```python
from build123d import *

# Parameters (mm, degrees)
SKETCH_2_W               = 1.6
SKETCH_2_H               = 0.7
CUT_EXTRUDE_1_DEPTH      = 3.5
CUT_EXTRUDE_1_DEPTH_BACK = 3.5
CHAMFER_1_SIZE           = 0.2


with BuildPart() as part:
    # 草图1 → 旋转1 (revolve)
    with BuildSketch(Plane(origin=(0, 0, 0), x_dir=(0, 0, -1), z_dir=(1, 0, 0))):
        Polygon((0, 0), (0, 2.5), (1.5, 2.5), (1.5, 1.5), (9.5, 1.5), (9.5, 0.7), (9.8, 0.7), (9.8, 1), (13.5, 1), (13.5, 0), align=None)
    revolve(axis=Axis((0, 0, -13.5), (0, 0, 1)))

    # 草图2 → 切除-拉伸1 (cut, two sides)
    with BuildSketch(Plane(origin=(0, 0, 0), x_dir=(0, 0, -1), z_dir=(1, 0, 0))) as cut_extrude_1_sk:
        Rectangle(SKETCH_2_W, SKETCH_2_H)
    extrude(amount=CUT_EXTRUDE_1_DEPTH, mode=Mode.SUBTRACT)
    extrude(cut_extrude_1_sk.sketch, amount=-CUT_EXTRUDE_1_DEPTH_BACK, mode=Mode.SUBTRACT)

    # 倒角1
    chamfer_1_edges = [part.edges().sort_by_distance(p)[0] for p in [
        (0, -2.5, 0),
        (-1.639359631, 1.887458609, 0),
    ]]
    chamfer(chamfer_1_edges, length=CHAMFER_1_SIZE)


solid = part.part
```
The model under review builds one solid part; all positions refer to its coordinate system, in mm. A direction names the side the tool comes from. Round coordinates to 2 decimals unless told otherwise and drop trailing zeros. Order: outer loops, then holes, each group sorted by start corner. A loop starts at its lowest first (then second) coordinate and runs counter-clockwise, first axis right, second up.
Item 1: Machinability: for faces 5 (the cylindrical face through (1, 0, -12)), 6 (the flat face through (0, 0, -13.5)), 7 (the flat face through (0, -0.35, -0.4)), which of the approach directions +Z, -Z, +X, -X, +Y, -Y give a long, thin tool a straight path to every point of the face, cutting with its end or side? Answer none if there is none.
Working result:
face 5: -Z
face 6: -Z, +X, -X, +Y, -Y
face 7: +Z, +X, -X
Item 2: Add section A-A, the plane y = 0. State the section outline as (x, z) points, and give its area (3 significant figures).
Working result:
outline: (-2.5, -1.5) - (-1.5, -1.5) - (-1.5, -9.5) - (-0.7, -9.5) - (-0.7, -9.8) - (-1, -9.8) - (-1, -13.5) - (1, -13.5) - (1, -9.8) - (0.7, -9.8) - (0.7, -9.5) - (1.5, -9.5) - (1.5, -1.5) - (2.5, -1.5) - (2.5, -0.8) - (-2.5, -0.8) - close
area: 35.3 mm2
Item 3: Add section C-C, the plane z = -10.75. State the section outline as (x, y) points.
Working result:
outline: circle Ø2 at (0, 0)
Item 4: Add section B-B, the plane x = 0. State the section outline as (y, z) points.
Working result:
outline: (-2.5, -1.5) - (-1.5, -1.5) - (-1.5, -9.5) - (-0.7, -9.5) - (-0.7, -9.8) - (-1, -9.8) - (-1, -13.5) - (1, -13.5) - (1, -9.8) - (0.7, -9.8) - (0.7, -9.5) - (1.5, -9.5) - (1.5, -1.5) - (2.5, -1.5) - (2.5, -0.2) - (2.3, 0) - (0.35, 0) - (0.35, -0.8) - (-0.35, -0.8) - (-0.35, 0) - (-2.3, 0) - (-2.5, -0.2) - close
Item 5: To check wall thickness, follow probe 1 along Z at (x, y) = (0.75, 1.9); probe 2 along X at (y, z) = (-0.05, -3.5); probe 3 along Z at (x, y) = (1, -0.85). State the ranges of each line that lie inside material, in increasing order.
Working result:
probe 1: z = -1.5 to 0
probe 2: x = -1.5 to 1.5
probe 3: z = -9.5 to 0
Item 6: Draft analysis for pull direction Z (two halves, no side actions). For faces 1 (the flat face through (0, 1, 0)), 2 (the flat face through (0, 1, -9.5)), 3 (the flat face through (0, 2, -1.5)), 4 (the cylindrical face through (-0.03, -0.7, -9.65)), state which applies: released by +Z, released by -Z, zero draft, split by the parting line, or undercut.
Working result:
face 1: released by +Z
face 2: undercut
face 3: released by -Z
face 4: undercut
Item 7: Add section D-D, the plane z = -7. State the section outline as (x, y) points.
Working result:
outline: circle Ø3 at (0, 0)
